The drawing under review shows one solid part. Ordinate dimensions are in mm from its lowest x, y, z. A direction names the side the tool comes from. Give positions to 0.01 mm unless a question says otherwise; leave off trailing zeros. Write each loop counter-clockwise with the first axis right and the second up, starting at its lowest first coordinate (ties: lowest second). Pieces come first, ordered by that corner, then holes. Notation, with made-up numbers: (1, -16) -> (28, -16) arc R12 ccw to (28, -9) -> close; hole circle Ø4 at (70.5, 28). An arc over 180 degrees is marked (long way). Use CSV: the item, a comma, the result in double quotes.
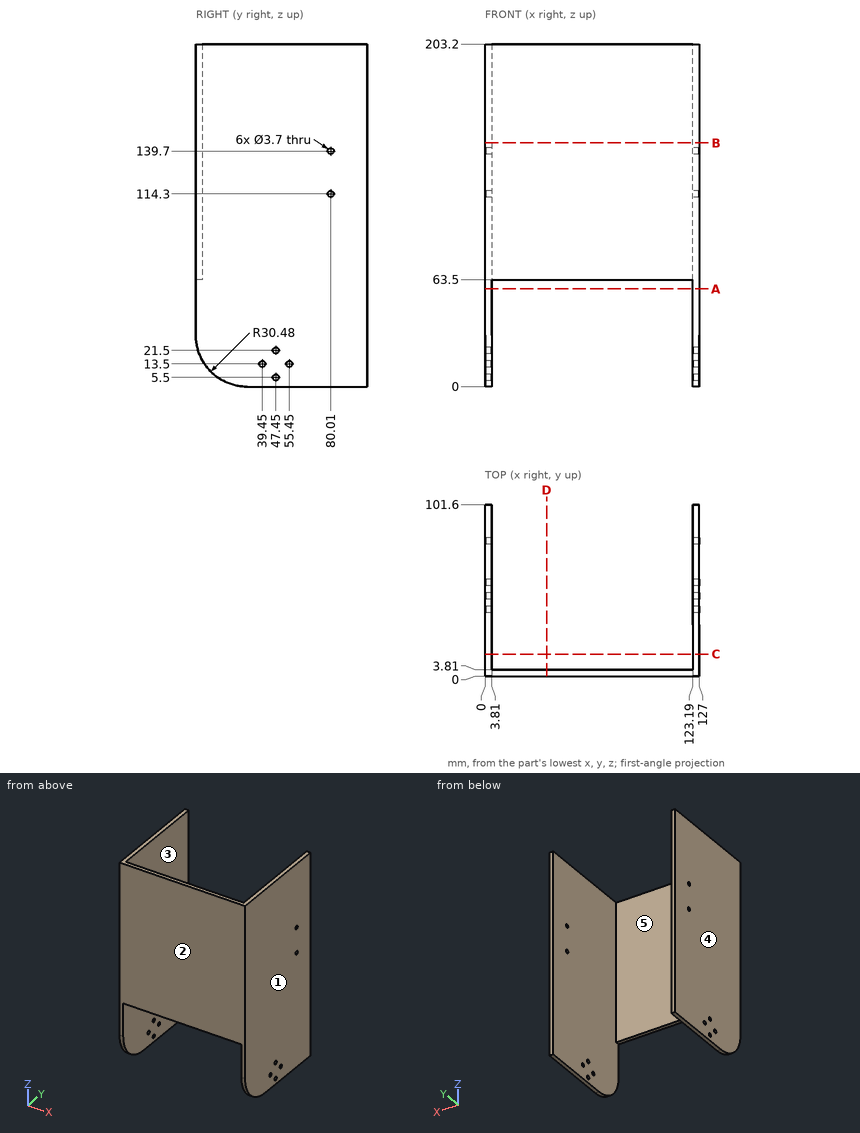
(1) Tool access review of the marked faces 4 and 5: name each direction out of +Z, -Z, +X, -X, +Y, -Y from which nothing blocks a thin tool from reaching the whole face with its end or side.
Established:
face 4,"+Z, -Z, -X, +Y, -Y"
face 5,"+Z, -Z, +Y"
(2) For line 1 along Z through (x, y) = (2.55, 47.45); line 2 along Z through (x, y) = (2.7, 80.01); line 3 along X through (y, z) = (39, 32), list the stretches that pass through material, from the lowest coordinate up. Write a range as [from, to].
Established:
line 1,"z = [0, 3.65], [7.35, 19.65], [23.35, 203.2]"
line 2,"z = [0, 112.45], [116.15, 137.85], [141.55, 203.2]"
line 3,"x = [0, 3.81], [123.19, 127]"
(3) Take a section at D-D (x = 36.5). Write out the cut boundary in (y, z), then the cut area to 3 significant figures.
Established:
outline,"(0, 63.5) -> (3.81, 63.5) -> (3.81, 203.2) -> (0, 203.2) -> close"
area,"532 mm2"
(4) Clearance check with flat-ended pins moving along their axes: pin 1 (2 mm diameter, centred on y = 55.45, z = 13.5, fed in from +X); pin 2 (6 mm diameter, centred on y = 39.45, z = 13.5, fed in from -X); pin 3 (2 mm diameter, centred on x = 103, z = 173.5, fed in from +Y); pin 4 (4 mm diameter, centred on x = 56, y = 2, fed in from -Z). State where each tip first meets the part, or that it passes through.
Established:
pin 1,"passes through"
pin 2,"stops at x = 0"
pin 3,"stops at y = 3.81"
pin 4,"stops at z = 63.5"
(5) Take a section at C-C (y = 13). Write out the cut boundary in (x, z), then the cut area to 3 significant figures.
Established:
outline,"(0, 5.51) -> (3.81, 5.51) -> (3.81, 203.2) -> (0, 203.2) -> close; (123.19, 5.51) -> (127, 5.51) -> (127, 203.2) -> (123.19, 203.2) -> close"
area,"1,510 mm2"
(6) Take a section at A-A (z = 58). Write out the cut boundary in (x, y), then the cut area to 3 significant figures.
Established:
outline,"(0, 0) -> (3.81, 0) -> (3.81, 101.6) -> (0, 101.6) -> close; (123.19, 0) -> (127, 0) -> (127, 101.6) -> (123.19, 101.6) -> close"
area,"774 mm2"
(7) Mouldability with a two-part tool opening along X and no side actions: class the marked faces 1, 2 and 3 as +X half, -X half, draft (parallel to the pull), parting line (faces both ways), or undercut.
Established:
face 1,"+X half"
face 2,"draft"
face 3,"undercut"
(8) Take a section at B-B (z = 144.5). Write out the cut boundary in (x, y).
Established:
outline,"(0, 0) -> (127, 0) -> (127, 101.6) -> (123.19, 101.6) -> (123.19, 3.81) -> (3.81, 3.81) -> (3.81, 101.6) -> (0, 101.6) -> close"
